from build123d import *

# Parameters (mm, degrees)
F1_DEPTH = 63.5
F2_DEPTH = 25.4
F3_DEPTH = 7.9375
F0_W     = 25.4
F0_H     = 19.05
F4_DEPTH = 25.4
F6_R     = 6.35


with BuildPart() as f1:
    # F0 (on Front) → F1 (new body, symmetric)
    with BuildSketch(Plane.XZ):
        Polygon((-41.275, -9.525), (41.275, -9.525), (41.275, 9.525), (22.225, 9.525), (-41.275, 9.525), align=None)
    extrude(amount=F1_DEPTH, both=True)

    # F0 (on Front) → F2 (join, symmetric)
    with BuildSketch(Plane.XZ):
        with BuildLine():
            Line((22.225, 9.525), (41.275, 9.525))
            Line((41.275, 9.525), (41.275, 27.0002))
            ThreePointArc((41.275, 27.0002), (45.9246798487, 38.2255201513), (57.15, 42.8752))
            Line((57.15, 42.8752), (60.325, 42.8752))
            Line((60.325, 42.8752), (60.325, 61.9252))
            Line((60.325, 61.9252), (57.15, 61.9252))
            add(Edge.make_bspline(
                [(54.9104785197, 61.8533227947), (55.6599311663, 61.8827305791), (56.4065455523, 61.9066982117), (57.15, 61.9252)],
                knots=[109.5628960552, 109.5628960552, 109.5628960552, 109.5628960552, 111.5045361635, 111.5045361635, 111.5045361635, 111.5045361635], degree=3))
            ThreePointArc((54.9104785197, 61.8533227947), (31.67480704, 50.8909967354), (22.225, 27.0002))
            Line((22.225, 27.0002), (22.225, 9.525))
        make_face()
    extrude(amount=F2_DEPTH, both=True)

    # F0 (on Front) → F3 (join, symmetric)
    with BuildSketch(Plane.XZ):
        with BuildLine():
            add(Edge.make_bspline(
                [(-41.275, 9.525), (-38.7071358638, 41.2123762099), (12.620353756, 60.1938999086), (54.9104785197, 61.8533227947)],
                knots=[0, 0, 0, 0, 109.5628960552, 109.5628960552, 109.5628960552, 109.5628960552], degree=3))
            Line((-41.275, 9.525), (22.225, 9.525))
            Line((22.225, 9.525), (22.225, 27.0002))
            ThreePointArc((22.225, 27.0002), (31.67480704, 50.8909967354), (54.9104785197, 61.8533227947))
        make_face()
    extrude(amount=F3_DEPTH, both=True)

    # F0 (on Front) → F4 (join, symmetric)
    with BuildSketch(Plane.XZ):
        with Locations((73.025, 52.4002)):
            Rectangle(F0_W, F0_H)
    extrude(amount=F4_DEPTH, both=True)

    # F0 (on Front) → F5 (revolve)
    with BuildSketch(Plane.XZ):
        Polygon((85.725, 61.9252), (85.725, 42.8752), (85.725, 38.1), (111.125, 38.1), (111.125, 66.675), (85.725, 66.675), align=None)
    revolve(axis=Axis((85.725, 0, 52.3875), (0, 0, 1)))

    # F6
    f6_edges = [f1.edges().sort_by_distance(p)[0] for p in [
        (-41.275, -63.5, 0),
        (41.275, -63.5, 0),
        (41.275, 63.5, 0),
        (-41.275, 63.5, 0),
    ]]
    fillet(f6_edges, radius=F6_R)


solid = f1.part
For this review, take the finished solid that the model builds, in its own axes (mm). A direction names the side the tool comes from. Coordinates: 2 decimals unless noted, no trailing zeros. Order: outer loops, then holes, each group sorted by start corner. A loop starts at its lowest first (then second) coordinate and runs counter-clockwise, first axis right, second up. Notation, with made-up numbers: (60, 84.25) -> (106, 84.25) arc R19 cw to (106, 99.25) -> close; hole circle Ø5 at (2, 59.5). An arc over 180 degrees is marked (long way). Return JSON: item names as keys, results as strings.
1. We need section B-B on x = 74.5. Write out the cut boundary in (y, z) (3 decimals).
Answer block:
{"outline": "(-25.4, 42.875) -> (-22.785, 42.875) -> (-22.785, 38.1) -> (22.785, 38.1) -> (22.785, 42.875) -> (25.4, 42.875) -> (25.4, 61.925) -> (22.785, 61.925) -> (22.785, 66.675) -> (-22.785, 66.675) -> (-22.785, 61.925) -> (-25.4, 61.925) -> close"}
2. Machinability: for faces 1 (the flat face through (-3, 7.938, 30)), 2 (the cylindrical face through (45.8, -0.4, 38.1)), 3 (the cylindrical face through (31.93, -16.79, 51.16)), which of the approach directions +Z, -Z, +X, -X, +Y, -Y give a long, thin tool a straight path to every point of the face, cutting with its end or side? Answer none if there is none.
Answer block:
{"face 1": "+Z, -X, +Y", "face 2": "-Z, +Y, -Y", "face 3": "+Z, -X, -Y"}
3. For line 1 (X direction, y = 20.5, z = 19.5) (3 decimals); line 2 (Z direction, x = -14, y = -51) (3 decimals); line 3 (X direction, y = 40.5, z = -3.5) (3 decimals), list the stretches that pass through material, from the lowest coordinate up. Write a range as from..to.
Answer block:
{"line 1": "22.225..41.275", "line 2": "-9.525..9.525", "line 3": "-41.275..41.275"}
4. We need section A-A on z = 1.5. Write out the cut boundary in (x, y) (3 decimals), and give its area (3 significant figures).
Answer block:
{"outline": "(-41.275, -57.15) arc R6.35 ccw to (-34.925, -63.5) -> (34.925, -63.5) arc R6.35 ccw to (41.275, -57.15) -> (41.275, 57.15) arc R6.35 ccw to (34.925, 63.5) -> (-34.925, 63.5) arc R6.35 ccw to (-41.275, 57.15) -> close", "area": "10,400 mm²"}
5. For pin 1 Ø4 at (y, z) = (8.5, 39) entering from +X; pin 2 Ø1 at (x, z) = (-15, 30.5) entering from -Y; pin 3 Ø15.5 at (x, z) = (59, 29.5) entering from -Y; pin 4 Ø5 at (y, z) = (-17, 39) entering from +X, all flat-tipped, find the tip position at first contact; note any pin that passes through.
Answer block:
{"pin 1": "x = 110.28", "pin 2": "y = -7.94", "pin 3": "through", "pin 4": "x = 106.58"}
